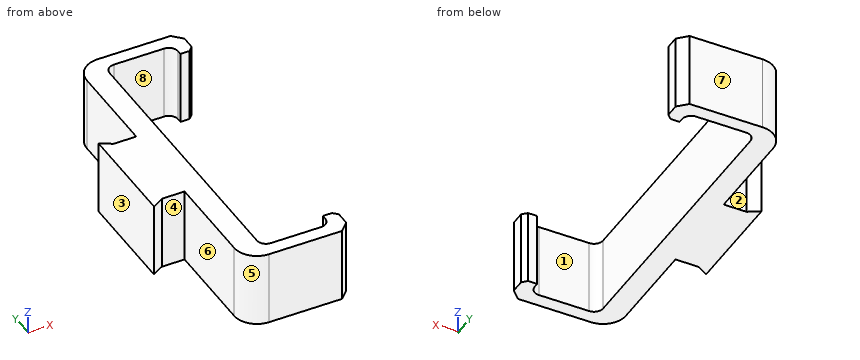
from build123d import *

# Parameters (mm, degrees)
F1_DEPTH = 16.5
F2_R     = 5
F3_R     = 2
F4_SIZE  = 1
F5_SIZE  = 2
F7_DEPTH = 16.5


with BuildPart() as f1:
    # F0 (on Top) → F1 (new body)
    with BuildSketch(Plane.XY):
        Polygon((23, 35.5), (0, 35.5), (0, 10), (-5, 10), (-5, -10), (0, -10), (0, -35.5), (23, -35.5), (23, -29.5), (20, -29.5), (20, -32.5), (5, -32.5), (5, 32.5), (20, 32.5), (20, 29.5), (23, 29.5), align=None)
    extrude(amount=F1_DEPTH)

    # F2
    f2_edges = [f1.edges().sort_by_distance(p)[0] for p in [
        (0, -35.5, 8.25),
        (0, 35.5, 8.25),
    ]]
    fillet(f2_edges, radius=F2_R)

    # F3
    f3_edges = [f1.edges().sort_by_distance(p)[0] for p in [
        (5, 32.5, 8.25),
        (5, -32.5, 8.25),
        (20, 32.5, 8.25),
        (20, -32.5, 8.25),
    ]]
    fillet(f3_edges, radius=F3_R)

    # F4
    f4_edges = [f1.edges().sort_by_distance(p)[0] for p in [
        (23, 29.5, 8.25),
        (23, -29.5, 8.25),
    ]]
    chamfer(f4_edges, length=F4_SIZE)

    # F5
    f5_edges = [f1.edges().sort_by_distance(p)[0] for p in [
        (23, 35.5, 8.25),
        (23, -35.5, 8.25),
    ]]
    chamfer(f5_edges, length=F5_SIZE)

    # F6 (on Top) → F7 (join)
    with BuildSketch(Plane.XY):
        Polygon((-5, 10), (-7.5, 11.5), (-7.5, -11.5), (-5, -10), align=None)
    extrude(amount=F7_DEPTH)


solid = f1.part
Model file for the job. Use its own axes, mm. Face numbers are marked on the shaded views. A direction names the side the tool comes from. Give positions to 0.01 mm unless a question says otherwise; leave off trailing zeros. Loops run counter-clockwise (first coordinate to the right, second up) from the corner with the lowest first, then second, coordinate; pieces in that order, holes last. Notation, with made-up numbers: (45.5, -19) -> (73.5, -19) arc R12 ccw to (73.5, -9) -> close; hole circle Ø6 at (80, 58.5). An arc over 180 degrees is marked (long way). Use a Markdown table: item, result. Add a question column.
(1) Slice it at C-C on x = 6. List the corners of the cut face in (y, z), and give its area (3 significant figures).
(2) Mould opens along Y. For the marked faces 6, 7 and 8 say: +Y half, -Y half, draft (parallel to the pull), parting line (faces both ways), or undercut.
(3) Drop flat-ended pins along their axis: pin 1 Ø2.5 at (x, z) = (-2, 6) entering from -Y; pin 2 Ø5 at (y, z) = (-22.5, 8) entering from -X; pin 3 Ø8 at (y, z) = (12.5, 10.5) entering from +X. Give the stop position or say it passes through.
(4) Tool access for the marked faces 1, 2, 3, 4 and 5: list every direction of +Z, -Z, +X, -X, +Y, -Y with a clear straight run to the whole face (end or side of a thin tool).
(5) Slice it at A-A on x = 12.5. List the corners of the cut face in (y, z), and give its area (3 significant figures).
(6) Wall check: line 1 along Y through (x, z) = (10.5, 13.25); line 2 along X through (y, z) = (13, 14.5); line 3 along Y through (x, z) = (-1.5, 4). Give the ranges that are in metal, low to high.
(7) Slice it at D-D on y = 6. List the corners of the cut face in (x, z), and give its area (3 significant figures).
(8) Slice it at B-B on z = 12.5. List the corners of the cut face in (x, y), and give its area (3 significant figures).
Filled sheet:
| question | item | result |
|---|---|---|
| 1 | outline | (-35.5, 0) -> (-32.23, 0) -> (-32.23, 16.5) -> (-35.5, 16.5) -> close; (32.23, 0) -> (35.5, 0) -> (35.5, 16.5) -> (32.23, 16.5) -> close |
| 1 | area | 108 mm2 |
| 2 | face 6 | draft |
| 2 | face 7 | +Y half |
| 2 | face 8 | undercut |
| 3 | pin 1 | y = -10 |
| 3 | pin 2 | x = 0 |
| 3 | pin 3 | x = 5 |
| 4 | face 1 | +Z, -Z |
| 4 | face 2 | +Z, -Z, +Y |
| 4 | face 3 | +Z, -Z, -X, +Y, -Y |
| 4 | face 4 | +Z, -Z, -Y |
| 4 | face 5 | +Z, -Z, -X, -Y |
| 5 | outline | (-35.5, 0) -> (-32.5, 0) -> (-32.5, 16.5) -> (-35.5, 16.5) -> close; (32.5, 0) -> (35.5, 0) -> (35.5, 16.5) -> (32.5, 16.5) -> close |
| 5 | area | 99.0 mm2 |
| 6 | line 1 | -35.5 to -32.5, 32.5 to 35.5 |
| 6 | line 2 | 0 to 5 |
| 6 | line 3 | -10 to 10 |
| 7 | outline | (-7.5, 0) -> (5, 0) -> (5, 16.5) -> (-7.5, 16.5) -> close |
| 7 | area | 206 mm2 |
| 8 | outline | (-7.5, -11.5) -> (-5, -10) -> (0, -10) -> (0, -30.5) arc R5 ccw to (5, -35.5) -> (21, -35.5) -> (23, -33.5) -> (23, -30.5) -> (22, -29.5) -> (20, -29.5) -> (20, -30.5) arc R2 cw to (18, -32.5) -> (7, -32.5) arc R2 cw to (5, -30.5) -> (5, 30.5) arc R2 cw to (7, 32.5) -> (18, 32.5) arc R2 cw to (20, 30.5) -> (20, 29.5) -> (22, 29.5) -> (23, 30.5) -> (23, 33.5) -> (21, 35.5) -> (5, 35.5) arc R5 ccw to (0, 30.5) -> (0, 10) -> (-5, 10) -> (-7.5, 11.5) -> close |
| 8 | area | 622 mm2 |
